Geometry check sheet. Reference: the model listing, model coordinates, mm. Face numbers are marked on the shaded views. A direction names the side the tool comes from. Round coordinates to 2 decimals unless told otherwise and drop trailing zeros. Write each loop counter-clockwise with the first axis right and the second up, starting at its lowest first coordinate (ties: lowest second). Pieces come first, ordered by that corner, then holes. Notation, with made-up numbers: (80.25, 4.25) -> (97.25, 4.25) arc R22 ccw to (97.25, 41.25) -> close; hole circle Ø5 at (-33.75, 79.25). An arc over 180 degrees is marked (long way). Return JSON: item names as keys, results as strings. Group by question number.
Autodesk Inventor part; units mm, degrees
ref_plane "YZ Plane" through (0, 0, 0) normal (1, 0, 0) x (0, 1, 0)
ref_plane "XZ Plane" through (0, 0, 0) normal (0, 1, 0) x (-1, 0, 0)
ref_plane "XY Plane" through (0, 0, 0) normal (0, 0, 1) x (1, 0, 0)
sketch "Sketch1" plane through (0, 0, 0) normal (0, 0, 1) x (1, 0, 0)
  line L0 (-9.4085, 11.4915) -> (2.7915, 11.4915)
  line L1 (2.7915, 11.4915) -> (2.7915, -10.5085)
  line L2 (2.7915, -10.5085) -> (-9.4085, -10.5085)
  line L3 (-9.4085, -10.5085) -> (-9.4085, 11.4915)
  point P0 (0, 0)
  dimension "d0" = 22
  dimension "d1" = 12.2
extrude "Extrusion1" add sketch "Sketch1" along normal blind 2
sketch "Sketch2" plane through (0, 0, 0) normal (0, 0, -1) x (-1, 0, 0)
  line L0 (-2.7915, -14.5085) -> (9.4085, -14.5085)
  line L1 (9.4085, -14.5085) -> (9.4085, 13.4915)
  line L2 (9.4085, 13.4915) -> (-2.7915, 13.4915)
  line L3 (-2.7915, 13.4915) -> (-2.7915, -14.5085)
  line L4 (9.4085, -10.5085) -> (9.4085, 11.4915)
  line L5 (-2.7915, 11.4915) -> (-2.7915, -10.5085)
  line L6 (9.4085, 11.4915) -> (-2.7915, 11.4915)
  line L7 (-2.7915, -10.5085) -> (9.4085, -10.5085)
  point P0 (0, 0)
  dimension "d4" = 2
  dimension "d5" = 4
extrude "Extrusion2" add sketch "Sketch2" along normal blind 0.4
sketch "Sketch3" plane through (2.7915, -10.5085, 2) normal (1, 0, 0) x (0, 0, -1)
  line L0 (0, 0) -> (0, 22)
  line L1 (2, 22) -> (0, 22)
  line L2 (2.4, 24) -> (2.4, -4)
  line L3 (2.4, 0) -> (11.7, 2)
  line L4 (11.7, 2) -> (9.9, 13.7)
  line L5 (9.9, 13.7) -> (2.4, 21.767)
  line L6 (2.4, 0) -> (2.4, 21.767)
  point P0 (2, 10.5085)
  dimension "d8" = 9.9
  dimension "d9" = 11.7
  dimension "d10" = 8.3
  dimension "d11" = 20
extrude "Extrusion3" add sketch "Sketch3" against normal blind 12
sketch "Sketch4" plane through (-9.2085, -10.5085, 2) normal (-1, 0, 0) x (0, 0, 1)
  line L0 (-2.4, -4) -> (-2.4, 24)
  line L1 (-2.4, 22) -> (-8.4, 22)
  line L2 (-8.4, 22) -> (-8.4, 3)
  line L3 (-8.4, 3) -> (-2.4, 3)
  line L4 (-2.4, 3) -> (-2.4, 22)
  line L5 (-2, 22) -> (0, 22)
  point P0 (-2, 10.5085)
  dimension "d14" = 6
  dimension "d15" = 19
extrude "Extrusion4" cut sketch "Sketch4" against normal blind 12
properties part number "button"
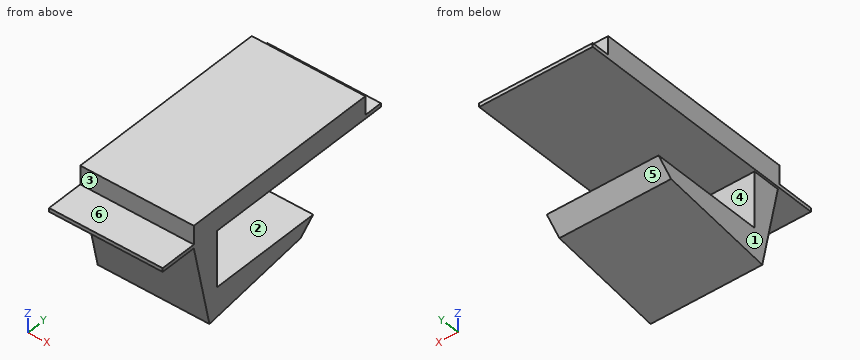
1) Tool access check on the marked faces 1, 2 and 3. Record the directions out of +Z, -Z, +X, -X, +Y, -Y that give a thin tool (end or side, any length) a straight path to the whole face; none if there is none.
2) Mould release check, pull along Z, two halves, no side actions. Record for the marked faces 4, 5 and 6: +Z half, -Z half, draft (parallel to the pull), parting line (faces both ways), or undercut.
3) Sectioned sample at D-D on y = -6.5. Enter the section's corners in (x, z), and give its area (3 significant figures).
4) Sectioned sample at B-B on y = 4. Enter the section's corners in (x, z), and give its area (3 significant figures).
5) Sectioned sample at C-C on z = 0.5. Enter the section's corners in (x, y), and give its area (3 significant figures).
6) Go/stop test with flat-tipped pins: P1, Ø5, axis at x = -1, z = -3, coming from the +Y side; P2, Ø0.6, axis at x = -0.5, z = 1, coming from the -Y side; P3, Ø3, axis at y = -4, z = -5.5, coming from the -X side. Record where each tip stops, or that it passes through.
7) Sectioned sample at A-A on x = -3.5. Enter the section's corners in (y, z).
8) Material ranges on probe 1 along Z at (x, y) = (-6.5, -12.5); probe 2 along X at (y, z) = (-10, -1.5); probe 3 along Z at (x, y) = (-2.75, 11.25), recorded low to high. Write a range as [from, to].
Evaluation:
{
 "1": {"face 1": "-Z, -X, +Y, -Y", "face 2": "+X, -X, +Y", "face 3": "+Z, +X, -X, -Y"},
 "2": {"face 4": "undercut", "face 5": "-Z half", "face 6": "+Z half"},
 "3": {"outline": "(-9.41, -0.4) -> (2.79, -0.4) -> (2.79, 2) -> (-9.41, 2) -> close; (-9.21, -9.39) -> (2.79, -9.39) -> (2.79, -6.4) -> (-9.21, -6.4) -> close", "area": "65.2 mm2"},
 "4": {"outline": "(-9.41, -0.4) -> (2.79, -0.4) -> (2.79, 2) -> (-9.41, 2) -> close; (-9.21, -7.15) -> (2.79, -7.15) -> (2.79, -6.4) -> (-9.21, -6.4) -> close", "area": "38.3 mm2"},
 "5": {"outline": "(-9.41, -10.51) -> (2.79, -10.51) -> (2.79, 11.49) -> (-9.41, 11.49) -> close", "area": "268 mm2"},
 "6": {"P1": "stops at y = -7.51", "P2": "stops at y = -10.51", "P3": "stops at x = -9.21"},
 "7": {"outline": "(-14.51, -0.4) -> (-10.51, -0.4) -> (-8.51, -9.7) -> (3.19, -7.9) -> (4.8, -6.4) -> (-7.51, -6.4) -> (-7.51, -0.4) -> (13.49, -0.4) -> (13.49, 0) -> (11.49, 0) -> (11.49, 2) -> (-10.51, 2) -> (-10.51, 0) -> (-14.51, 0) -> close"},
 "8": {"probe 1": "z = [-0.4, 0]", "probe 2": "x = [-9.21, 2.79]", "probe 3": "z = [-0.4, 2]"}
}
